Could you check a few things on this model? Use its own coordinates, in mm. Round coordinates to 2 decimals unless told otherwise and drop trailing zeros. Loops run counter-clockwise (first coordinate to the right, second up) from the corner with the lowest first, then second, coordinate; pieces in that order, holes last. Notation, with made-up numbers: (45, 31.25) -> (80, 31.25) arc R6 cw to (80, 40.25) -> close; hole circle Ø8 at (27.5, 43.5). An arc over 180 degrees is marked (long way). Write each question's results on one line, items separated by ' | '.
from build123d import *

# Parameters (mm, degrees)
SKETCH1_R      = 3.5814
SKETCH1_R_2    = 0.7112
SKETCH1_R_3    = 2.38125
EXTRUDE1_DEPTH = 0.8255


with BuildPart() as part:
    # Sketch1 → Extrude1 (new body, symmetric)
    with BuildSketch(Plane(origin=(0, 0, 0), x_dir=(1, 0, 0), z_dir=(0, 1, 0))):
        with BuildLine():
            Line((3.914177728, 12.720888158), (5.880660619, 0.985406368))
            ThreePointArc((5.880660619, 0.985406368), (0, -5.96265), (-5.880660619, 0.985406368))
            Line((-5.880660619, 0.985406368), (-3.914177728, 12.720888158))
            ThreePointArc((-3.914177728, 12.720888158), (0, 16.03375), (3.914177728, 12.720888158))
        make_face()
        with Locations(Location((0, 0, 0), (0, 0, 270))):  # turned: the seam where the file's is
            Circle(SKETCH1_R, mode=Mode.SUBTRACT)
        with Locations(Location((0, 4.8514, 0), (0, 0, 270))):  # turned: the seam where the file's is
            Circle(SKETCH1_R_2, mode=Mode.SUBTRACT)
        with Locations(Location((0, 6.6802, 0), (0, 0, 270))):  # turned: the seam where the file's is
            Circle(SKETCH1_R_2, mode=Mode.SUBTRACT)
        with Locations(Location((0, 8.509, 0), (0, 0, 270))):  # turned: the seam where the file's is
            Circle(SKETCH1_R_2, mode=Mode.SUBTRACT)
        with Locations(Location((0, 12.065, 0), (0, 0, 270))):  # turned: the seam where the file's is
            Circle(SKETCH1_R_3, mode=Mode.SUBTRACT)
    extrude(amount=EXTRUDE1_DEPTH, both=True)


solid = part.part
1) I need wall thicknesses on line 1 (Z direction, x = 2, y = 0.3); line 2 (Z direction, x = 1.25, y = 0.35); line 3 (X direction, y = -0.25, z = 0). Which ranges of each line are inside material? Lowest first, please.
Model answer:
line 1: z = -15.49 to -13.36, -10.77 to -2.97, 2.97 to 5.62 | line 2: z = -15.83 to -14.09, -10.04 to -3.36, 3.36 to 5.83 | line 3: x = -5.96 to -3.58, 3.58 to 5.96
2) I'm going to push a flat-ended pin straight in: pin 1 (1.1 mm diameter, centred on x = 0, z = -4.85, fed in from +Y). Where does the tip first touch, or does it pass through?
Model answer:
pin 1: passes through
3) I want a section at B-B, the plane x = 0. Write out the boundary of the cut face in (y, z), plus the area to 3 significant figures.
Model answer:
outline: (-0.83, -16.03) -> (0.83, -16.03) -> (0.83, -14.45) -> (-0.83, -14.45) -> close; (-0.83, -9.68) -> (0.83, -9.68) -> (0.83, -9.22) -> (-0.83, -9.22) -> close; (-0.83, -7.8) -> (0.83, -7.8) -> (0.83, -7.39) -> (-0.83, -7.39) -> close; (-0.83, -5.97) -> (0.83, -5.97) -> (0.83, -5.56) -> (-0.83, -5.56) -> close; (-0.83, -4.14) -> (0.83, -4.14) -> (0.83, -3.58) -> (-0.83, -3.58) -> close; (-0.83, 3.58) -> (0.83, 3.58) -> (0.83, 5.96) -> (-0.83, 5.96) -> close | area: 9.58 mm2
4) I want a section at A-A, the plane z = 0. Write out the boundary of the cut face in (x, y), plus the area to 3 significant figures.
Model answer:
outline: (-5.96, -0.83) -> (-3.58, -0.83) -> (-3.58, 0.83) -> (-5.96, 0.83) -> close; (3.58, -0.83) -> (5.96, -0.83) -> (5.96, 0.83) -> (3.58, 0.83) -> close | area: 7.86 mm2
5) I want a section at C-C, the plane y = 0.4. Write out the boundary of the cut face in (x, z) (1 decimal).
Model answer:
outline: (-5.9, -1) -> (-3.9, -12.7) arc R4 ccw to (3.9, -12.7) -> (5.9, -1) arc R6 ccw (long way) to start; hole circle Ø7.2 at (0, 0); hole circle Ø4.8 at (0, -12.1); hole circle Ø1.4 at (0, -8.5); hole circle Ø1.4 at (0, -6.7); hole circle Ø1.4 at (0, -4.9)
6) If we mould it in two halves opening along Z, with no side actions, what happens to faces 1 (the cylindrical face through (0.21, -0.01, -4.17)), 2 (the flat face through (-4.91, 0.01, -6.77)), 3 (the flat face through (-1, -0.826, -5))? For each: released by +Z, released by -Z, zero draft, split by the parting line, or undercut.
Model answer:
face 1: undercut | face 2: released by -Z | face 3: zero draft
7) I want a section at D-D, the plane x = 1.75. Write out the boundary of the cut face in (y, z).
Model answer:
outline: (-0.83, -15.63) -> (0.83, -15.63) -> (0.83, -13.68) -> (-0.83, -13.68) -> close; (-0.83, -10.45) -> (0.83, -10.45) -> (0.83, -3.12) -> (-0.83, -3.12) -> close; (-0.83, 3.12) -> (0.83, 3.12) -> (0.83, 5.7) -> (-0.83, 5.7) -> close
